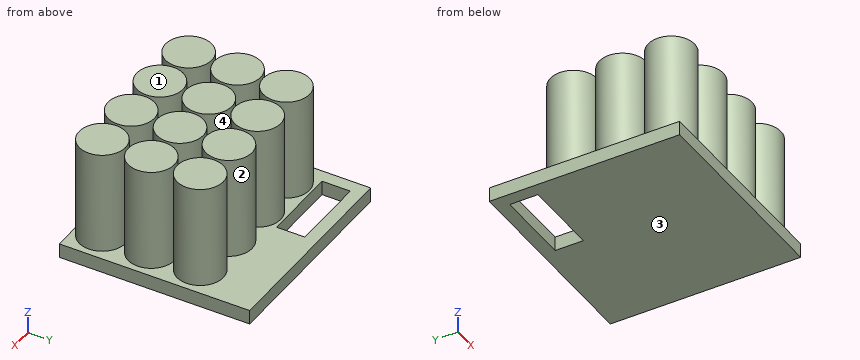
from build123d import *

# Parameters (mm, degrees)
SKETCH_1_W      = 80
SKETCH_1_H      = 74
SKETCH_1_W_2    = 30
SKETCH_1_H_2    = 11
EXTRUDE_1_DEPTH = 5.6
SKETCH_2_R      = 9
EXTRUDE_2_DEPTH = 40


with BuildPart() as part:
    # 草图1 → 凸台-拉伸1 (new body)
    with BuildSketch(Plane.XY):
        with Locations((4.975124378, -23.343283582)):
            Rectangle(SKETCH_1_W, SKETCH_1_H)
        with Locations((-15.024875622, 3.156716418)):
            Rectangle(SKETCH_1_W_2, SKETCH_1_H_2, mode=Mode.SUBTRACT)
    extrude(amount=-EXTRUDE_1_DEPTH)

    # 草图2 → 凸台-拉伸2 (add)
    with BuildSketch(Plane.XY):
        with Locations((-23.524875622, -50.343283582)):
            Circle(SKETCH_2_R)
        with Locations((-4.524875622, -50.343283582)):
            Circle(SKETCH_2_R)
        with Locations((14.475124378, -50.343283582)):
            Circle(SKETCH_2_R)
        with Locations((33.475124378, -50.343283582)):
            Circle(SKETCH_2_R)
        with Locations((-4.524875622, -31.343283582)):
            Circle(SKETCH_2_R)
        with Locations((14.475124378, -31.343283582)):
            Circle(SKETCH_2_R)
        with Locations((33.475124378, -31.343283582)):
            Circle(SKETCH_2_R)
        with Locations((-4.524875622, -12.343283582)):
            Circle(SKETCH_2_R)
        with Locations((14.475124378, -12.343283582)):
            Circle(SKETCH_2_R)
        with Locations((33.475124378, -12.343283582)):
            Circle(SKETCH_2_R)
        with Locations((-23.524875622, -31.343283582)):
            Circle(SKETCH_2_R)
        with Locations((-23.524875622, -12.343283582)):
            Circle(SKETCH_2_R)
    extrude(amount=EXTRUDE_2_DEPTH)


solid = part.part
Geometry: final body of the model. Coordinates: model frame, mm. Face numbers are marked on the shaded views. A direction names the side the tool comes from. Round coordinates to 2 decimals unless told otherwise and drop trailing zeros. Loops run counter-clockwise (first coordinate to the right, second up) from the corner with the lowest first, then second, coordinate; pieces in that order, holes last. Notation, with made-up numbers: M -1,22.25 L 47,22.25 A33 ccw 47,61.25 Z; hole C 54.25,-30.5 d1. An arc over 180 degrees is marked long. Put each result on its own line as item: value. Start each with the question number.
(1) Section query C-C (z = 4.5). State how many separate pieces and enclosed holes the cut face has, then the cut area to 3 significant figures.
(2) Contact query for flat-ended pins moving along their axis: pin 1 Ø4 at (x, z) = (33.5, 28) entering from -Y; pin 2 Ø2 at (x, z) = (7, 27.5) entering from +Y; pin 3 Ø3 at (x, z) = (36.5, 29.5) entering from +Y. Output: stop coordinate, or through.
(3) Section query B-B (x = -6.5). Return loops of the section in (y, z), then the cut area to 3 significant figures.
(4) Section query D-D (y = -47.5). Return loops of the section in (x, z).
(5) Section query A-A (z = -1). Return loops of the section in (x, y).
(6) Material intervals for line 1 along Y through (x, z) = (-23, 21); line 2 along Y through (x, z) = (-10, 28); line 3 along X through (y, z) = (-27.5, 15), sorted ascending. Write a range as [from, to].
(7) Set-up query: the marked faces 3 and 4. Return all of +Z, -Z, +X, -X, +Y, -Y with unobstructed straight access to the full face (end or side cutting, diameter ignored); none if empty.
(8) Draft query along X for the marked faces 1 and 2. Return one class per face: +X half, -X half, draft (parallel to the pull), parting line (faces both ways), or undercut.
Findings below:
1. separate pieces: 12
1. enclosed holes: 0
1. area: 3,050 mm2
2. pin 1: stops at y = -59.34
2. pin 2: stops at y = -6.09
2. pin 3: stops at y = -3.47
3. outline: M -60.34,-5.6 L -2.34,-5.6 L -2.34,0 L -3.56,0 L -3.56,40 L -21.12,40 L -21.12,0 L -22.56,0 L -22.56,40 L -40.12,40 L -40.12,0 L -41.56,0 L -41.56,40 L -59.12,40 L -59.12,0 L -60.34,0 Z; M 8.66,-5.6 L 13.66,-5.6 L 13.66,0 L 8.66,0 Z
3. area: 2,460 mm2
4. outline: M -35.02,-5.6 L 44.98,-5.6 L 44.98,0 L 42.01,0 L 42.01,40 L 24.94,40 L 24.94,0 L 23.01,0 L 23.01,40 L 5.94,40 L 5.94,0 L 4.01,0 L 4.01,40 L -13.06,40 L -13.06,0 L -14.99,0 L -14.99,40 L -32.06,40 L -32.06,0 L -35.02,0 Z
5. outline: M -35.02,-60.34 L 44.98,-60.34 L 44.98,13.66 L -35.02,13.66 Z; hole M -30.02,-2.34 L -0.02,-2.34 L -0.02,8.66 L -30.02,8.66 Z
6. line 1: y = [-59.33, -41.36], [-40.33, -22.36], [-21.33, -3.36]
6. line 2: y = [-57.49, -43.2], [-38.49, -24.2], [-19.49, -5.2]
6. line 3: x = [-31.66, -15.39], [-12.66, 3.61], [6.34, 22.61], [25.34, 41.61]
7. face 3: -Z, +X, -X, +Y, -Y
7. face 4: +Z
8. face 1: draft
8. face 2: undercut
